Could you check a few things on this model? Use its own coordinates, in mm. A direction names the side the tool comes from. Give positions to 0.01 mm unless a question says otherwise; leave off trailing zeros. Order: outer loops, then holes, each group sorted by start corner. A loop starts at its lowest first (then second) coordinate and runs counter-clockwise, first axis right, second up. Notation, with made-up numbers: (52.25, 12) -> (78.25, 12) arc R24 ccw to (78.25, 41) -> close; hole circle Ø5 at (83, 17.5). An arc over 180 degrees is marked (long way). Answer as CSV lines item,"result". Start each with the question number.
(1) I need wall thicknesses on L1, parallel to X at y = -124, z = 4.15; L2, parallel to Y at x = 109, z = 1.15; L3, parallel to Y at x = 237, z = 2.5. Which ranges of each line are inside material? Lowest first, please.
(2) I want a section at A-A (x = 184). Please give me the cut outline in (y, z), plus the area to 3 significant figures.
(3) Will these pins go through, and if not, where does the flat tip stop? pin 1 Ø2.5 at (y, z) = (-120.5, 3.5) entering from +X; pin 2 Ø1 at (x, z) = (223.5, 1.5) entering from -Y; pin 3 Ø1.5 at (x, y) = (57, -34) entering from -Z.
(4) On a 3-axis mill with a long thin cutter (end or side, diameter ignored), from which of +Z, -Z, +X, -X, +Y, -Y can I reach the whole of each face in a straight line? I mean faces 1 (the face through (126.52, -151.35, 2.54)), 2 (the face through (123, -83, 5)). Say none if no direction works.
(5) I want a section at C-C (y = -119.5). Please give me the cut outline in (x, z).
(6) We'd pull the mould along Y, two halves only. Please class faces 3 (the face through (5, -128, 3)), 4 (the face through (36, -98, 3)), 5 (the face through (123, -83, 0)), 6 (the face through (147, -217.428, 3)): released by +Y, released by -Y, zero draft, split by the parting line, or undercut.
(7) I want a section at D-D (x = 59). Please give me the cut outline in (y, z).
(8) I want a section at B-B (z = 4.05). Please give me the cut outline in (x, y), plus the area to 3 significant figures.
```python
from build123d import *

# Parameters (mm, degrees)
SKETCH1_W           = 249.6
SKETCH1_H           = 267.4
BOSS_EXTRUDE1_DEPTH = 5
CUT_EXTRUDE3_DEPTH  = 6


with BuildPart() as part:
    # Sketch1 → Boss-Extrude1 (new body)
    with BuildSketch(Plane.XY):
        with Locations((124.8, -133.7)):
            Rectangle(SKETCH1_W, SKETCH1_H)
    extrude(amount=BOSS_EXTRUDE1_DEPTH)

    # Sketch5 → Cut-Extrude3 (cut, through all)
    with BuildSketch(Plane.XY.offset(5)):
        with BuildLine():
            Line((124.8, -267.4), (249.6, -267.4))
            Line((249.6, -267.4), (249.6, -99.925464159))
            ThreePointArc((249.6, -99.925464159), (175.224742578, -139.824828971), (208.410715021, -217.428498098))
            Line((208.410715021, -217.428498098), (83.524571607, -217.428498098))
            ThreePointArc((83.524571607, -217.428498098), (126.353700731, -150.143883017), (66, -98))
            Line((66, -98), (5, -98))
            Line((5, -98), (5, -159))
            ThreePointArc((5, -159), (17.061268569, -195.414290683), (48.475428393, -217.428498098))
            Line((48.475428393, -217.428498098), (0, -217.428498098))
            Line((0, -217.428498098), (0, -267.4))
            Line((0, -267.4), (124.8, -267.4))
        make_face()
    extrude(amount=-CUT_EXTRUDE3_DEPTH, mode=Mode.SUBTRACT)


solid = part.part
```
Final values:
1,L1,"0 to 5, 115.96 to 183.47"
1,L2,"-217.43 to -202.27, -115.73 to 0"
1,L3,"-98.06 to 0"
2,outline,"(-217.43, 0) -> (-197.72, 0) -> (-197.72, 5) -> (-217.43, 5) -> close; (-123.28, 0) -> (0, 0) -> (0, 5) -> (-123.28, 5) -> close"
2,area,"715 mm²"
3,pin 1,"x = 187.25"
3,pin 2,"y = -99.01"
3,pin 3,"z = 0"
4,face 1,"+Z, -Z"
4,face 2,"+Z, +X, -X, +Y, -Y"
5,outline,"(0, 0) -> (5, 0) -> (5, 5) -> (0, 5) -> close; (112.48, 0) -> (187.03, 0) -> (187.03, 5) -> (112.48, 5) -> close"
6,face 3,"undercut"
6,face 4,"undercut"
6,face 5,"zero draft"
6,face 6,"released by -Y"
7,outline,"(-98, 0) -> (0, 0) -> (0, 5) -> (-98, 5) -> close"
8,outline,"(0, -217.43) -> (48.48, -217.43) arc R61 cw to (5, -159) -> (5, -98) -> (66, -98) arc R61 cw to (83.52, -217.43) -> (208.41, -217.43) arc R62.5 cw to (249.6, -99.93) -> (249.6, 0) -> (0, 0) -> close"
8,area,"34,000 mm²"
